```python
from build123d import *

# Parameters (mm, degrees)
SKETCH1_R           = 5.3975
BOSS_EXTRUDE1_DEPTH = 5.08
SKETCH3_R           = 3.5306
BOSS_EXTRUDE2_DEPTH = 3.175
SKETCH4_R           = 4.7625
BOSS_EXTRUDE3_DEPTH = 6.985
CHAMFER1_SIZE       = 1.27
CHAMFER2_SIZE       = 1.27


with BuildPart() as part:
    # Sketch1 → Boss-Extrude1 (new body)
    with BuildSketch(Plane.XY):
        Circle(SKETCH1_R)
    extrude(amount=BOSS_EXTRUDE1_DEPTH)

    # Sketch3 → Boss-Extrude2 (add)
    with BuildSketch(Plane.XY.offset(5.08)):
        Circle(SKETCH3_R)
    extrude(amount=BOSS_EXTRUDE2_DEPTH)

    # Sketch4 → Boss-Extrude3 (add)
    with BuildSketch(Plane.XY.offset(8.255)):
        Circle(SKETCH4_R)
    extrude(amount=BOSS_EXTRUDE3_DEPTH)

    # Chamfer1
    chamfer1_edges = [part.edges().sort_by_distance(p)[0] for p in [
        (-4.7625, 0, 15.24),
    ]]
    chamfer(chamfer1_edges, length=CHAMFER1_SIZE)

    # Chamfer2
    chamfer2_edges = [part.edges().sort_by_distance(p)[0] for p in [
        (-5.3975, 0, 0),
    ]]
    chamfer(chamfer2_edges, length=CHAMFER2_SIZE)


solid = part.part
```
Here's how the part is built. I have some questions about the finished solid (model axes, mm). A direction names the side the tool comes from. Coordinates: 2 decimals unless noted, no trailing zeros. Write each loop counter-clockwise with the first axis right and the second up, starting at its lowest first coordinate (ties: lowest second). Pieces come first, ordered by that corner, then holes. Notation, with made-up numbers: (19.25, 26.5) -> (64.25, 26.5) arc R11 cw to (64.25, 34.5) -> close; hole circle Ø3 at (-12, 55). An arc over 180 degrees is marked (long way). Use a Markdown table: item, result. Add a question column.
(1) We'd pull the mould along Z, two halves only. Please class faces 3 (the flat face through (0, 0, 15.24)), 4 (the cylindrical face through (-3.978, 3.648, 3.148)), 5 (the flat face through (1, -4, 5.08)), 6 (the flat face through (0, 0, 0)): +Z half, -Z half, draft (parallel to the pull), parting line (faces both ways), or undercut.
(2) Please list where these lines run through material, in increasing order: line 1 (Z direction, x = 3.5, y = -3) (3 decimals); line 2 (Z direction, x = 1.5, y = 4.25) (3 decimals); line 3 (X direction, y = 5, z = 4).
(3) If we section it at C-C, the plane z = 8.5: Write out the boundary of the cut face in (x, y) (1 decimal), and give its area (3 significant figures).
(4) For faces 1 (the flat face through (-4, 0, 8.255)), 2 (the cylindrical face through (-3.78, -2.9, 11.07)), which set-ups out of +Z, -Z, +X, -X, +Y, -Y let a thin tool reach every point of the face, with its end or its side?
(5) If we section it at D-D, the plane z = 3.5: Write out the boundary of the cut face in (x, y) (1 decimal), and give its area (3 significant figures).
(6) I'm going to push flat-ended pins straight in: P1, Ø3, axis at y = -3, z = 2.5, coming from the +X side; P2, Ø1.5, axis at x = 1, z = 11.5, coming from the -Y side; P3, Ø5, axis at x = -3.5, z = 3, coming from the -Y side. Where does each tip first touch, or does it pass through?
(7) If we section it at A-A, the plane y = 0: Write out the boundary of the cut face in (x, z) (1 decimal).
Outcome:
| question | item | result |
|---|---|---|
| 1 | face 3 | +Z half |
| 1 | face 4 | draft |
| 1 | face 5 | undercut |
| 1 | face 6 | -Z half |
| 2 | line 1 | z = 0.482 to 5.08, 8.255 to 14.123 |
| 2 | line 2 | z = 0.379 to 5.08, 8.255 to 14.226 |
| 2 | line 3 | x = -2.03 to 2.03 |
| 3 | outline | circle Ø9.5 at (0, 0) |
| 3 | area | 71.3 mm^2 |
| 4 | face 1 | none |
| 4 | face 2 | +Z |
| 5 | outline | circle Ø10.8 at (0, 0) |
| 5 | area | 91.5 mm^2 |
| 6 | P1 | stops at x = 5.18 |
| 6 | P2 | stops at y = -4.76 |
| 6 | P3 | stops at y = -5.3 |
| 7 | outline | (-5.4, 1.3) -> (-4.1, 0) -> (4.1, 0) -> (5.4, 1.3) -> (5.4, 5.1) -> (3.5, 5.1) -> (3.5, 8.3) -> (4.8, 8.3) -> (4.8, 14) -> (3.5, 15.2) -> (-3.5, 15.2) -> (-4.8, 14) -> (-4.8, 8.3) -> (-3.5, 8.3) -> (-3.5, 5.1) -> (-5.4, 5.1) -> close |
